Work out the finished part from the listing and answer in its coordinate system (mm). A direction names the side the tool comes from. Give positions to 0.01 mm unless a question says otherwise; leave off trailing zeros. Order: outer loops, then holes, each group sorted by start corner. A loop starts at its lowest first (then second) coordinate and runs counter-clockwise, first axis right, second up.
```python
from build123d import *

# Parameters (mm, degrees)
SKETCH1_W           = 30
SKETCH1_H           = 25
SKETCH1_R           = 1.75
BOSS_EXTRUDE1_DEPTH = 5
BOSS_EXTRUDE2_DEPTH = 5
SKETCH3_W           = 19.5
SKETCH3_H           = 5
BOSS_EXTRUDE3_DEPTH = 30
SKETCH4_R           = 1.75
CUT_EXTRUDE1_DEPTH  = 32
FILLET1_R           = 5
FILLET2_R           = 2


with BuildPart() as part:
    # Sketch1 → Boss-Extrude1 (new body)
    with BuildSketch(Plane(origin=(0, 0, 0), x_dir=(1, 0, 0), z_dir=(0, 1, 0))):
        Rectangle(SKETCH1_W, SKETCH1_H)
        with Locations((-10, -2.5)):
            Circle(SKETCH1_R, mode=Mode.SUBTRACT)
        with Locations((10, -2.5)):
            Circle(SKETCH1_R, mode=Mode.SUBTRACT)
    extrude(amount=BOSS_EXTRUDE1_DEPTH)

    # Sketch2 → Boss-Extrude2 (add)
    with BuildSketch(Plane.ZY.offset(15)):
        Polygon((-12.5, 5), (12.5, 5), (12.5, 0), (-7.5, 0), (-7.5, -21), (12.5, -21), (12.5, -26), (-12.5, -26), align=None)
    extrude(amount=BOSS_EXTRUDE2_DEPTH)

    # Sketch3 → Boss-Extrude3 (add)
    with BuildSketch(Plane(origin=(-15, 0, 0), x_dir=(0, 0, -1), z_dir=(1, 0, 0))):
        with Locations((-2.75, -23.5)):
            Rectangle(SKETCH3_W, SKETCH3_H)
    extrude(amount=BOSS_EXTRUDE3_DEPTH)

    # Sketch4 → Cut-Extrude1 (cut, through all)
    with BuildSketch(Plane.XZ.offset(26)):
        with Locations((-10, 2.5)):
            Circle(SKETCH4_R)
        with Locations((10, 2.5)):
            Circle(SKETCH4_R)
    extrude(amount=-CUT_EXTRUDE1_DEPTH, mode=Mode.SUBTRACT)

    # Fillet1
    fillet1_edges = [part.edges().sort_by_distance(p)[0] for p in [
        (-17.5, -26, -12.5),
        (15, -23.5, -7),
        (15, 2.5, -12.5),
    ]]
    fillet(fillet1_edges, radius=FILLET1_R)

    # Fillet2
    fillet2_edges = [part.edges().sort_by_distance(p)[0] for p in [
        (-20, -8, -12.5),
        (-20, 5, 0),
        (15, -26, 5.25),
        (15, 5, 2.5),
        (-2.5, -26, -7),
        (-20, -26, 2.5),
        (13.535533906, -26, -5.535533906),
        (-5, 5, -12.5),
        (-20, -24.535533906, -11.035533906),
        (13.535533906, 5, -11.035533906),
    ]]
    fillet(fillet2_edges, radius=FILLET2_R)


solid = part.part
```
1. The part is cut by section B-B (z = -0.75). Write down the section's boundary in (x, y), then the cut area to 3 significant figures.
Findings below:
outline: (-20, -24) arc R2 ccw to (-18, -26) - (13, -26) arc R2 ccw to (15, -24) - (15, -21) - (-20, -21) - close; (-20, 0) - (15, 0) - (15, 3) arc R2 ccw to (13, 5) - (-18, 5) arc R2 ccw to (-20, 3) - close
area: 347 mm2
2. The part is cut by section D-D (z = 2.5). Write down the section's boundary in (x, y), then the cut area to 3 significant figures.
Findings below:
outline: (-20, -24) arc R2 ccw to (-18, -26) - (-11.75, -26) - (-11.75, -21) - (-20, -21) - close; (-20, 0) - (-11.75, 0) - (-11.75, 5) - (-18, 5) arc R2 ccw to (-20, 3) - close; (-8.25, -26) - (8.25, -26) - (8.25, -21) - (-8.25, -21) - close; (-8.25, 0) - (8.25, 0) - (8.25, 5) - (-8.25, 5) - close; (11.75, -26) - (13, -26) arc R2 ccw to (15, -24) - (15, -21) - (11.75, -21) - close; (11.75, 0) - (15, 0) - (15, 3) arc R2 ccw to (13, 5) - (11.75, 5) - close
area: 277 mm2
3. The part is cut by section C-C (x = -14.5). Write down the section's boundary in (y, z), then the cut area to 3 significant figures.
Findings below:
outline: (-26, -5) arc R2 ccw to (-24, -7) - (-21, -7) - (-21, 12.5) - (-26, 12.5) - close; (0, -12.5) - (3, -12.5) arc R2 ccw to (5, -10.5) - (5, 12.5) - (0, 12.5) - close
area: 221 mm2
4. The mould has two halves that part along Z. Classify faces 1 (the face through (11.617, 2.465, 3.17)), 2 (the face through (-3, -24, 12.5)), 3 (the face through (-8.383, -23.535, 1.83)), 4 (the face through (15, 1, 3)): pulls with the +Z half, pulls with the -Z half, needs draft (parallel to the pull), parting line crosses it, or undercut.
Findings below:
face 1: undercut
face 2: pulls with the +Z half
face 3: undercut
face 4: needs draft
5. The part is cut by section A-A (x = -10). Write down the section's boundary in (y, z).
Findings below:
outline: (-26, -5) arc R2 ccw to (-24, -7) - (-21, -7) - (-21, 0.75) - (-26, 0.75) - close; (-26, 4.25) - (-21, 4.25) - (-21, 12.5) - (-26, 12.5) - close; (0, -12.5) - (3, -12.5) arc R2 ccw to (5, -10.5) - (5, 0.75) - (0, 0.75) - close; (0, 4.25) - (5, 4.25) - (5, 12.5) - (0, 12.5) - close
6. Which of the six approach directions +Z, -Z, +X, -X, +Y, -Y give full straight-line access (tool end or side, diameter ignored) to faces 5 (the face through (-15, -13, -10)), 6 (the face through (-19.43, -25.4, 2.36)), 7 (the face through (-17, -10, -7.5))?
Findings below:
face 5: -Z, +X, -Y
face 6: +Z, -Z, -X, -Y
face 7: +Z, +X, -X
7. Straight lines are drawn through the part: probe 1 along X at (y, z) = (1.9, 2.5); probe 2 along Y at (x, z) = (5.5, 5.25); probe 3 along Z at (x, y) = (-10, -22.05). For each, find the intervals that lie inside material, in ascending order.
Findings below:
probe 1: x = -20 to -11.75, -8.25 to 8.25, 11.75 to 15
probe 2: y = -26 to -21, 0 to 5
probe 3: z = -7 to 0.75, 4.25 to 12.5
8. Given P1, Ø8, axis at x = 11, y = -18.5, coming from the -Z side; P2, Ø4, axis at y = -15, z = -8.5, coming from the +X side; P3, Ø1.5, axis at x = -17.5, y = -14.5, coming from the +Z side; P4, Ø3, axis at x = -10, z = 2.5, coming from the +Y side, each flat-ended and moving along its own axis, determine where each tip first touches the part or whether it passes through.
Findings below:
P1: stops at z = -7
P2: stops at x = -15
P3: stops at z = -7.5
P4: passes through
